```python
from build123d import *

# Parameters (mm, degrees)
SALIENTE_EXTRUIR1_DEPTH = 3
CORTAR_EXTRUIR1_DEPTH   = 3


with BuildPart() as part:
    # Croquis1 → Saliente-Extruir1 (new body)
    with BuildSketch(Plane(origin=(0, 0, 0), x_dir=(0, 0, -1), z_dir=(1, 0, 0))):
        Polygon((-46.517058898, 28.196284567), (53.482941102, 28.196284567), (53.482941102, 3.196284567), (56.482941102, 3.196284567), (56.482941102, -21.803715433), (53.482941102, -21.803715433), (53.482941102, -46.803715433), (56.482941102, -46.803715433), (56.482941102, -71.803715433), (53.482941102, -71.803715433), (53.482941102, -96.803715433), (-46.517058898, -96.803715433), (-46.517058898, -71.803715433), (-49.517058898, -71.803715433), (-49.517058898, -46.803715433), (-46.517058898, -46.803715433), (-46.517058898, -21.803715433), (-49.517058898, -21.803715433), (-49.517058898, 3.196284567), (-46.517058898, 3.196284567), align=None)
    extrude(amount=SALIENTE_EXTRUIR1_DEPTH)

    # Croquis2 → Cortar-Extruir1 (cut)
    with BuildSketch(Plane(origin=(3, 0, 0), x_dir=(0, 0, -1), z_dir=(1, 0, 0))):
        with BuildLine():
            Line((-6.517058898, -90.803715433), (-6.517058898, -84.803715433))
            ThreePointArc((-6.517058898, -84.803715433), (-4.517058898, -82.803715433), (-2.517058898, -84.803715433))
            Line((-2.517058898, -84.803715433), (-2.517058898, -90.803715433))
            ThreePointArc((-2.517058898, -90.803715433), (-4.517058898, -92.803715433), (-6.517058898, -90.803715433))
        make_face()
        with BuildLine():
            Line((13.482941102, -90.803715433), (13.482941102, -84.803715433))
            ThreePointArc((13.482941102, -84.803715433), (11.482941102, -82.803715433), (9.482941102, -84.803715433))
            Line((9.482941102, -84.803715433), (9.482941102, -90.803715433))
            ThreePointArc((9.482941102, -90.803715433), (11.482941102, -92.803715433), (13.482941102, -90.803715433))
        make_face()
    extrude(amount=-CORTAR_EXTRUIR1_DEPTH, mode=Mode.SUBTRACT)


solid = part.part
```
CAD build for the part. Positions are in the model's coordinates, mm. A direction names the side the tool comes from. Round coordinates to 2 decimals unless told otherwise and drop trailing zeros. Loops run counter-clockwise (first coordinate to the right, second up) from the corner with the lowest first, then second, coordinate; pieces in that order, holes last. Notation, with made-up numbers: (69.5, -38) - (119.5, -38) arc R22 cw to (119.5, -27) - close; hole circle Ø11 at (19, -31.75). An arc over 180 degrees is marked (long way). Return JSON: item names as keys, results as strings. Group by question number.
Q1. Flat gauge pins, fed straight in: pin 1 Ø1.5 at (x, y) = (1, -33) entering from +Z; pin 2 Ø1.5 at (x, z) = (2, 48) entering from +Y; pin 3 Ø0.9 at (x, z) = (2, 48.5) entering from -Y; pin 4 Ø10 at (y, z) = (-33, -32) entering from -X. Where does each tip first touch, or does it go through?
Q2. Band-saw the part on A-A on x = 1.15. Give the cut face in (y, z).
Q3. Band-saw the part on B-B on y = -88.5. Give the cut face in (x, z), plus the area to 3 significant figures.
Q4. Tool access for faces 1 (the face through (1, -34, -53.483)), 2 (the face through (1, 16, 46.517)), 3 (the face through (1.521, -82.804, -11.527)): list every direction of +Z, -Z, +X, -X, +Y, -Y with a clear straight run to the whole face (end or side of a thin tool).
Q5. Two-plate mould, pull along Z, no slides. Class faces 4 (the face through (1.521, -82.804, 4.561)), 5 (the face through (1, -59, -56.483)), 6 (the face through (3, -33, -4)): +Z half, -Z half, draft (parallel to the pull), parting line (faces both ways), or undercut.
Q6. Drill centre lines: line 1 along Z through (x, y) = (0.75, -87); line 2 along Z through (x, y) = (0.9, 17.5). Where is each one in solid material? Low to high. Write a range as [from, to].
Q7. Band-saw the part on C-C on y = 10. Give the cut face in (x, z).
Solutions:
{
 "1": {"pin 1": "stops at z = 46.52", "pin 2": "stops at y = 3.2", "pin 3": "stops at y = -71.8", "pin 4": "stops at x = 0"},
 "2": {"outline": "(-96.8, -53.48) - (-71.8, -53.48) - (-71.8, -56.48) - (-46.8, -56.48) - (-46.8, -53.48) - (-21.8, -53.48) - (-21.8, -56.48) - (3.2, -56.48) - (3.2, -53.48) - (28.2, -53.48) - (28.2, 46.52) - (3.2, 46.52) - (3.2, 49.52) - (-21.8, 49.52) - (-21.8, 46.52) - (-46.8, 46.52) - (-46.8, 49.52) - (-71.8, 49.52) - (-71.8, 46.52) - (-96.8, 46.52) - close; hole (-90.8, -13.48) - (-84.8, -13.48) arc R2 ccw to (-84.8, -9.48) - (-90.8, -9.48) arc R2 ccw to start; hole (-90.8, 2.52) - (-84.8, 2.52) arc R2 ccw to (-84.8, 6.52) - (-90.8, 6.52) arc R2 ccw to start"},
 "3": {"outline": "(0, -53.48) - (3, -53.48) - (3, -13.48) - (0, -13.48) - close; (0, -9.48) - (3, -9.48) - (3, 2.52) - (0, 2.52) - close; (0, 6.52) - (3, 6.52) - (3, 46.52) - (0, 46.52) - close", "area": "276 mm^2"},
 "4": {"face 1": "-Z, +X, -X", "face 2": "+Z, +X, -X, +Y", "face 3": "+X, -X"},
 "5": {"face 4": "undercut", "face 5": "-Z half", "face 6": "draft"},
 "6": {"line 1": "z = [-53.48, -13.48], [-9.48, 2.52], [6.52, 46.52]", "line 2": "z = [-53.48, 46.52]"},
 "7": {"outline": "(0, -53.48) - (3, -53.48) - (3, 46.52) - (0, 46.52) - close"}
}
